Verification items for the finished model (mm, model axes). A direction names the side the tool comes from. Give positions to 0.01 mm unless a question says otherwise; leave off trailing zeros. Write each loop counter-clockwise with the first axis right and the second up, starting at its lowest first coordinate (ties: lowest second). Pieces come first, ordered by that corner, then holes.
from build123d import *

# Parameters (mm, degrees)
SKETCH1_W                   = 50.8
SKETCH1_H                   = 50.8
SKETCH1_W_2                 = 44.45
SKETCH1_H_2                 = 44.45
BOSS_EXTRUDE1_DEPTH         = 495.3
FILLET1_R                   = 6.35
CUT_EXTRUDE1_DEPTH          = 914.4
F_1_2_CLEARANCE_HOLE1_D     = 13.49248
F_3_4_START                 = -25.4
F_3_4_CLEARANCE_SLOT1_DEPTH = 50.8


# Read off the part's stored shape, not the designer's step: 3/4 Clearance Slot1
with BuildPart() as part:
    # Sketch1 → Boss-Extrude1 (new, symmetric)
    with BuildSketch(Plane.XY):
        Rectangle(SKETCH1_W, SKETCH1_H)
        Rectangle(SKETCH1_W_2, SKETCH1_H_2, mode=Mode.SUBTRACT)
    extrude(amount=BOSS_EXTRUDE1_DEPTH, both=True)

    # Fillet1
    fillet1_edges = [part.edges().sort_by_distance(p)[0] for p in [
        (-25.4, 25.4, 0),
        (25.4, 25.4, 0),
        (25.4, -25.4, 0),
        (-25.4, -25.4, 0),
    ]]
    fillet(fillet1_edges, radius=FILLET1_R)

    # Sketch2 → Cut-Extrude1 (cut)
    with BuildSketch(Plane.ZY.offset(25.4)):
        Polygon((495.3, -25.4), (444.5, 25.4), (495.3, 25.4), align=None)
        Polygon((-495.3, 25.4), (-495.3, -25.4), (-444.5, 25.4), align=None)
    extrude(amount=-CUT_EXTRUDE1_DEPTH, mode=Mode.SUBTRACT)

    # 1/2 Clearance Hole1 (through all)
    with Locations(Plane.ZY.offset(25.4)):
        with Locations((-171.45, 0), (-311.15, 0), (-31.75, 0)):
            Hole(F_1_2_CLEARANCE_HOLE1_D / 2)

    # 3/4 Clearance Slot1 outline → 3/4 Clearance Slot1 (cut)
    with BuildSketch(Plane(origin=(0, 0, 0), x_dir=(1, 0, 0), z_dir=(0, 1, 0)).offset(F_3_4_START)):
        with BuildLine():
            ThreePointArc((9.72312, 129.97688), (0, 139.7), (-9.72312, 129.97688))
            Line((-9.72312, 129.97688), (-9.72312, 111.32312))
            ThreePointArc((-9.72312, 111.32312), (0, 101.6), (9.72312, 111.32312))
            Line((9.72312, 111.32312), (9.72312, 129.97688))
        make_face()
    extrude(amount=F_3_4_CLEARANCE_SLOT1_DEPTH, mode=Mode.SUBTRACT)


solid = part.part
Item 1: Sectioned sample at A-A on z = 249.5. Record the cut outline in (x, y) (3 decimals), then the cut area to 3 significant figures.
Answer key:
outline: (-25.4, -19.05) arc R6.35 ccw to (-19.05, -25.4) - (19.05, -25.4) arc R6.35 ccw to (25.4, -19.05) - (25.4, 19.05) arc R6.35 ccw to (19.05, 25.4) - (-19.05, 25.4) arc R6.35 ccw to (-25.4, 19.05) - close; hole (-22.225, -22.225) - (22.225, -22.225) - (22.225, 22.225) - (-22.225, 22.225) - close
area: 570 mm2
Item 2: Set-up check for faces 5 (the face through (22.225, 0, 7)), 6 (the face through (22.5, -0.1, 470)): record each of +Z, -Z, +X, -X, +Y, -Y from which the full face is reachable in a straight line by a thin tool's end or side.
Answer key:
face 5: +Z, -Z
face 6: +Z, +X, -X, +Y
Item 3: Depth check by flat-ended pin: pin 1 (11 mm diameter, centred on y = 0, z = -31.75, fed in from -X); pin 2 (3.5 mm diameter, centred on y = 24.5, z = -124, fed in from +X); pin 3 (3.5 mm diameter, centred on y = -24.5, z = -121, fed in from -X); pin 4 (12 mm diameter, centred on x = -17, y = -10.5, fed in from +Z). Enter the tip coordinate at first touch or a pass-through.
Answer key:
pin 1: passes through
pin 2: stops at x = 24.21
pin 3: stops at x = -24.21
pin 4: stops at z = 483.35
Item 4: Sectioned sample at B-B on x = 0. Record the cut outline in (y, z) (3 decimals), then the cut area to 3 significant figures.
Answer key:
outline: (-25.4, -495.3) - (-22.225, -492.125) - (-22.225, -139.7) - (-25.4, -139.7) - close; (-25.4, -101.6) - (-22.225, -101.6) - (-22.225, 492.125) - (-25.4, 495.3) - close; (22.225, -447.675) - (25.4, -444.5) - (25.4, -139.7) - (22.225, -139.7) - close; (22.225, -101.6) - (25.4, -101.6) - (25.4, 444.5) - (22.225, 447.675) - close
area: 5,730 mm2
Item 5: Scan lines: line 1 along X through (y, z) = (-9.5, -124.5) (3 decimals); line 2 along Y through (x, z) = (10, 448) (3 decimals). Record each from-to range of solid material in increasing order.
Answer key:
line 1: x = -25.4 to -22.225, 22.225 to 25.4
line 2: y = -25.4 to -22.225
Item 6: Release check for a two-part mould opening along X. For faces 1 (the face through (0, 22.225, 6)), 2 (the face through (-25.4, 0, 7)), 3 (the face through (0, 25.4, 6)), 4 (the face through (0, -22.225, 7)) record: released by +X, released by -X, zero draft, split by the parting line, or undercut.
Answer key:
face 1: undercut
face 2: released by -X
face 3: zero draft
face 4: undercut
